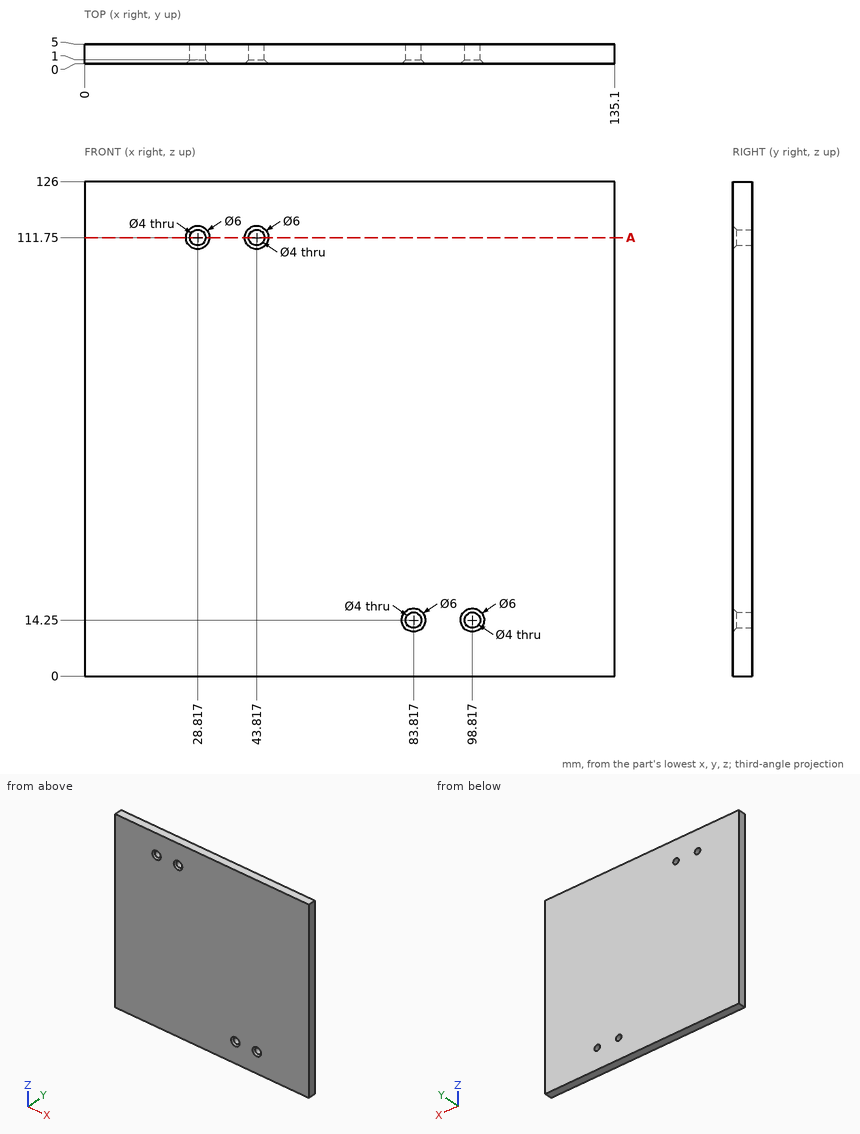
Input: dimensioned drawing with shaded views. Units: mm. Origin: part minimum x, y, z. Coordinates: 2 decimals unless noted, no trailing zeros. Order: outer loops, then holes, each group sorted by start corner. A loop starts at its lowest first (then second) coordinate and runs counter-clockwise, first axis right, second up. Notation, with made-up numbers: M 6.25,20 L 25.25,20 A28 ccw 25.25,46 Z; hole C 81.5,15.5 d11. An arc over 180 degrees is marked long. Answer as CSV lines item,"result".
Q1. First-contact query: P1, Ø4.5, axis at x = 98.817, z = 14.25, coming from the -Y side. Flat tip, straight axial feed; report the tip coordinate or a pass-through.
Answers:
P1,"stops at y = 0.75"
Q2. Section A-A on z = 111.75. Return the cut outline in (x, y), and give its area (4 significant figures).
Answers:
outline,"M 0,0 L 25.82,0 L 26.82,1 L 26.82,5 L 0,5 Z; M 30.82,1 L 31.82,0 L 40.82,0 L 41.82,1 L 41.82,5 L 30.82,5 Z; M 45.82,1 L 46.82,0 L 135.1,0 L 135.1,5 L 45.82,5 Z"
area,"633.5 mm^2"
Q3. Line query: probe 1 along X at (y, z) = (2.35, 14.25); probe 2 along X at (y, z) = (2.6, 111.75). Output: solid intervals per line, ascending. Write a range as [from, to].
Answers:
probe 1,"x = [0, 81.82], [85.82, 96.82], [100.82, 135.1]"
probe 2,"x = [0, 26.82], [30.82, 41.82], [45.82, 135.1]"
